```python
from build123d import *

# Parameters (mm, degrees)
SKIZZE1_W                            = 44
SKIZZE1_H                            = 25
AUFSATZ_LINEAR_AUSTRAGEN1_DEPTH      = 6.5
SKIZZE2_R                            = 5.675
SCHNITT_LINEAR_AUSTRAGEN1_DEPTH      = 5.1
VERRUNDUNG1_R                        = 2
SKIZZE8_W                            = 5.8
SKIZZE8_H                            = 2.6
SCHNITT_LINEAR_AUSTRAGEN5_DEPTH      = 4.5
SCHNITT_LINEAR_AUSTRAGEN6_DEPTH      = 2.6
SCHNITT_LINEAR_AUSTRAGEN7_DEPTH      = 31.698697041
SCHNITT_LINEAR_AUSTRAGEN7_DEPTH_BACK = 4.1
FASE1_SIZE                           = 0.5


with BuildPart() as part:
    # Skizze1 → Aufsatz-Linear austragen1 (new body)
    with BuildSketch(Plane.XY):
        with Locations((0, -2.5)):
            Rectangle(SKIZZE1_W, SKIZZE1_H)
    extrude(amount=AUFSATZ_LINEAR_AUSTRAGEN1_DEPTH)

    # Skizze2 → Schnitt-Linear austragen1 (cut)
    with BuildSketch(Plane.XY.offset(6.5)):
        Circle(SKIZZE2_R)
    extrude(amount=-SCHNITT_LINEAR_AUSTRAGEN1_DEPTH, mode=Mode.SUBTRACT)

    # Verrundung1
    verrundung1_edges = [part.edges().sort_by_distance(p)[0] for p in [
        (-22, 10, 3.25),
        (22, 10, 3.25),
        (22, -15, 3.25),
        (-22, -15, 3.25),
    ]]
    fillet(verrundung1_edges, radius=VERRUNDUNG1_R)

    # Skizze8 → Schnitt-Linear austragen5 (cut)
    with BuildSketch(Plane.XY.offset(6.5)):
        with Locations((0, -11.7)):
            Rectangle(SKIZZE8_W, SKIZZE8_H)
    extrude(amount=-SCHNITT_LINEAR_AUSTRAGEN5_DEPTH, mode=Mode.SUBTRACT)

    # Skizze9 → Schnitt-Linear austragen6 (cut)
    with BuildSketch(Plane.XZ.offset(10.4)):
        with BuildLine():
            Line((-0.820441954, 2), (-2.775, 2))
            Line((-2.775, 2), (0, 0.397853003))
            Line((0, 0.397853003), (2.775, 2))
            Line((2.775, 2), (0.820441954, 2))
            ThreePointArc((0.820441954, 2), (0, 1.802146997), (-0.820441954, 2))
        make_face()
        with BuildLine():
            ThreePointArc((1.8, 3.602146997), (-0.938936761, 5.137854573), (-0.820441954, 2))
            Line((-0.820441954, 2), (0.820441954, 2))
            ThreePointArc((0.820441954, 2), (1.535707576, 2.663210236), (1.8, 3.602146997))
        make_face()
        with BuildLine():
            Line((0.820441954, 2), (-0.820441954, 2))
            ThreePointArc((-0.820441954, 2), (0, 1.802146997), (0.820441954, 2))
        make_face()
    extrude(amount=SCHNITT_LINEAR_AUSTRAGEN6_DEPTH, mode=Mode.SUBTRACT)

    # Skizze9<3> → Schnitt-Linear austragen7 (cut, two sides: drawn at the far end of the back side and taken through both)
    with BuildSketch(Plane.XZ.offset(10.4).offset(-SCHNITT_LINEAR_AUSTRAGEN7_DEPTH_BACK)):
        with BuildLine():
            ThreePointArc((1.8, 3.602146997), (-0.938936761, 5.137854573), (-0.820441954, 2))
            Line((-0.820441954, 2), (0.820441954, 2))
            ThreePointArc((0.820441954, 2), (1.535707576, 2.663210236), (1.8, 3.602146997))
        make_face()
        with BuildLine():
            Line((0.820441954, 2), (-0.820441954, 2))
            ThreePointArc((-0.820441954, 2), (0, 1.802146997), (0.820441954, 2))
        make_face()
    extrude(amount=SCHNITT_LINEAR_AUSTRAGEN7_DEPTH + SCHNITT_LINEAR_AUSTRAGEN7_DEPTH_BACK, mode=Mode.SUBTRACT)

    # Fase1
    fase1_edges = [part.edges().sort_by_distance(p)[0] for p in [
        (-5.675, 0, 6.5),
        (0, 10, 0),
        (0, 10, 6.5),
        (-22, -2.5, 0),
        (22, -2.5, 0),
        (0, -15, 0),
        (-21.414213562, -14.414213562, 0),
        (-21.414213562, 9.414213562, 0),
        (21.414213562, -14.414213562, 0),
        (21.414213562, 9.414213562, 0),
        (22, -2.5, 6.5),
        (-22, -2.5, 6.5),
        (0, -15, 6.5),
        (-21.414213562, -14.414213562, 6.5),
        (-21.414213562, 9.414213562, 6.5),
        (21.414213562, -14.414213562, 6.5),
        (21.414213562, 9.414213562, 6.5),
        (2.9, -11.7, 6.5),
        (0, -10.4, 6.5),
        (-2.9, -11.7, 6.5),
        (0, -13, 6.5),
    ]]
    chamfer(fase1_edges, length=FASE1_SIZE)


solid = part.part
```
Build history of the part. All positions in model axes, mm. A direction names the side the tool comes from. Round coordinates to 2 decimals unless told otherwise and drop trailing zeros. Loops run counter-clockwise (first coordinate to the right, second up) from the corner with the lowest first, then second, coordinate; pieces in that order, holes last. Notation, with made-up numbers: M 45.25,43 L 77.25,43 A12 ccw 77.25,60 Z; hole C 37.25,29 d10. An arc over 180 degrees is marked long. Answer as CSV lines item,"result".
1. Cut at A-A on y = 0. Write the cut outline in (x, z) (3 decimals), then the cut area to 3 significant figures.
Resolved:
outline,"M -22,0.5 L -21.5,0 L 21.5,0 L 22,0.5 L 22,6 L 21.5,6.5 L 6.175,6.5 L 5.675,6 L 5.675,1.4 L -5.675,1.4 L -5.675,6 L -6.175,6.5 L -21.5,6.5 L -22,6 Z"
area,"227 mm²"
2. Two-plate mould, pull along Y, no slides. Class faces 4 (the conical face through (21.17, -14.15, 6.36)), 5 (the cylindrical face through (-21.43, 9.4, 3.29)), 6 (the flat face through (-1.41, -11.68, 1.21)): released by +Y, released by -Y, zero draft, split by the parting line, or undercut.
Resolved:
face 4,"released by -Y"
face 5,"released by +Y"
face 6,"undercut"
3. Cut at B-B on z = 4.5. Write the cut outline in (x, y) (3 decimals).
Resolved:
outline,"M -22,-13 A2 ccw -20,-15 L -1.56,-15 L -1.56,-13 L -2.9,-13 L -2.9,-10.4 L -1.56,-10.4 L -1.56,-6.3 L 1.56,-6.3 L 1.56,-10.4 L 2.9,-10.4 L 2.9,-13 L 1.56,-13 L 1.56,-15 L 20,-15 A2 ccw 22,-13 L 22,8 A2 ccw 20,10 L -20,10 A2 ccw -22,8 Z; hole C 0,0 d11.35"
4. Wall check: probe 1 along Y at (x, z) = (0, 4.5) (3 decimals); probe 2 along X at (y, z) = (-12, 5.25); probe 3 along X at (y, z) = (-4.5, 3.75). Give the ranges that are in metal, low to high. Write a range as [from, to].
Resolved:
probe 1,"y = [-6.3, -5.675], [5.675, 10]"
probe 2,"x = [-22, -2.9], [2.9, 22]"
probe 3,"x = [-22, -3.46], [3.46, 22]"
5. Flat gauge pins, fed straight in: P1, Ø9, axis at x = 0.5, y = -1, coming from the +Z side; P2, Ø1.5, axis at x = -0.5, z = 3, coming from the -Y side; P3, Ø3, axis at x = -0.5, z = 3, coming from the -Y side. Where does each tip first touch, or does it go through?
Resolved:
P1,"stops at z = 1.4"
P2,"stops at y = -6.3"
P3,"stops at y = -15"
6. 3-axis set-ups, long thin cutter, end or side, ignore diameter. For faces 1 (the flat face through (0, -6.3, 4)), 2 (the flat face through (0, 0, 1.4)), 3 (the conical face through (21.15, 9.17, 6.36)): which of +Z, -Z, +X, -X, +Y, -Y reach the whole face in a straight line?
Resolved:
face 1,"-Y"
face 2,"+Z"
face 3,"+Z, +X, +Y"
